Check sheet for the modelled part. Datum: model origin and axes. Units: mm. Face numbers are marked on the shaded views. A direction names the side the tool comes from. Round coordinates to 2 decimals unless told otherwise and drop trailing zeros. Write each loop counter-clockwise with the first axis right and the second up, starting at its lowest first coordinate (ties: lowest second). Pieces come first, ordered by that corner, then holes. Notation, with made-up numbers: (-30, 8.25) -> (-7, 8.25) arc R16 ccw to (-7, 26.25) -> close; hole circle Ø5 at (32, 49). An arc over 180 degrees is marked (long way). Answer as a JSON object with one key per item and string values. Group by question number.
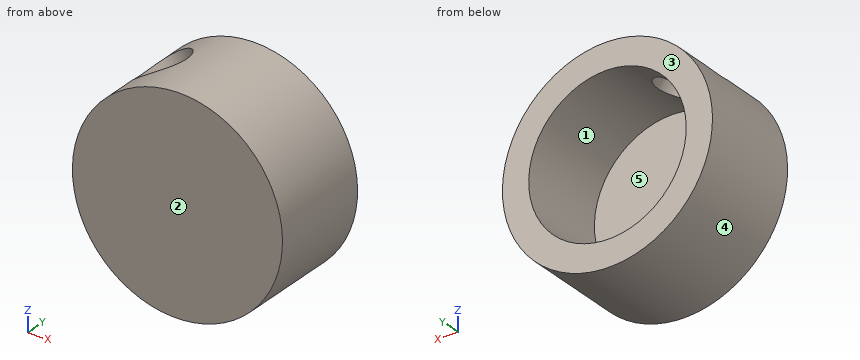
```python
from build123d import *

# Parameters (mm, degrees)
SKETCH_1_R                   = 40
EXTRUDE_1_DEPTH              = 40
SKETCH_3_R                   = 30
CUT_EXTRUDE_2_DEPTH          = 35
HOLE_WIZARD_21_0_21_1_REACH  = 100.524
HOLE_WIZARD_21_0_21_1_BORE_R = 10.5


with BuildPart() as part:
    # 草圖1 → 填料-伸長1 (new body)
    with BuildSketch(Plane(origin=(0, 0, 0), x_dir=(1, 0, 0), z_dir=(0, 1, 0))):
        with Locations(Location((0, 0, 0), (0, 0, 270))):
            Circle(SKETCH_1_R)
    extrude(amount=EXTRUDE_1_DEPTH)

    # 草圖3 → 除料-伸長2 (cut)
    with BuildSketch(Plane(origin=(0, 40, 0), x_dir=(1, 0, 0), z_dir=(0, 1, 0))):
        with Locations(Location((0, 0, 0), (0, 0, 270))):
            Circle(SKETCH_3_R)
    extrude(amount=-CUT_EXTRUDE_2_DEPTH, mode=Mode.SUBTRACT)

    # Ø21.0 (21) 直徑孔1 bore (on position points) → Ø21.0 (21) 直徑孔1 (cut, up to next)
    with BuildSketch(Plane(origin=(-21.744758151, 21.94181737, 33.573285406), x_dir=(0.839332135156, 0, 0.543618953768), z_dir=(-0.543618953768, 0, 0.839332135156)), mode=Mode.PRIVATE) as hole_wizard_21_0_21_1_sk1:
        Circle(HOLE_WIZARD_21_0_21_1_BORE_R)
    hole_wizard_21_0_21_1_tool1 = extrude(hole_wizard_21_0_21_1_sk1.sketch, amount=-HOLE_WIZARD_21_0_21_1_REACH, mode=Mode.PRIVATE) & part.part
    add(hole_wizard_21_0_21_1_tool1.solids().sort_by_distance((-21.744758, 21.941817, 33.573285))[0], mode=Mode.SUBTRACT)


solid = part.part
```
(1) Section check C-C on y = 8.5. Record the cut outline in (x, z), then the cut area to 3 significant figures.
(2) Section check D-D on y = 2. Record the cut outline in (x, z).
(3) Release check for a two-part mould opening along Z. For the marked faces 3, 4 and 5 record: pulls with the +Z half, pulls with the -Z half, needs draft (parallel to the pull), parting line crosses it, or undercut.
(4) Section check A-A on z = 0. Record the cut outline in (x, y).
(5) Section check B-B on x = 0. Record the cut outline in (y, z).
(6) Access from +Z, -Z, +X, -X, +Y, -Y to the whole of each face (thin tool, end or side, straight path). Record for the marked faces 1 and 2.
(7) Scan lines: line 1 along X through (y, z) = (18, 0); line 2 along X through (y, z) = (8, 10); line 3 along Z through (x, y) = (-8, 9.5). Record each from-to range of solid material in increasing order.
(8) Go/stop test with flat-tipped pins: pin 1 Ø18 at (x, z) = (-11, 11.5) entering from +Y; pin 2 Ø3 at (y, z) = (31.5, 30) entering from +X; pin 3 Ø8 at (y, z) = (22.5, -20.5) entering from +X. Record where each tip stops, or that it passes through.
Data:
{
 "1": {"outline": "circle Ø80 at (0, 0); hole circle Ø60 at (0, 0)", "area": "2,200 mm²"},
 "2": {"outline": "circle Ø80 at (0, 0)"},
 "3": {"face 3": "needs draft", "face 4": "parting line crosses it", "face 5": "undercut"},
 "4": {"outline": "(-40, 0) -> (40, 0) -> (40, 40) -> (30, 40) -> (30, 5) -> (-30, 5) -> (-30, 40) -> (-40, 40) -> close"},
 "5": {"outline": "(0, -40) -> (40, -40) -> (40, -30) -> (5, -30) -> (5, 30) -> (40, 30) -> (40, 40) -> (0, 40) -> close"},
 "6": {"face 1": "+Y", "face 2": "+Z, -Z, +X, -X, -Y"},
 "7": {"line 1": "x = -40 to -30, 30 to 40", "line 2": "x = -38.73 to -28.28, 28.28 to 38.73", "line 3": "z = -39.19 to -28.91, 28.91 to 39.19"},
 "8": {"pin 1": "stops at y = 5", "pin 2": "stops at x = 28.07", "pin 3": "stops at x = 36.44"}
}
